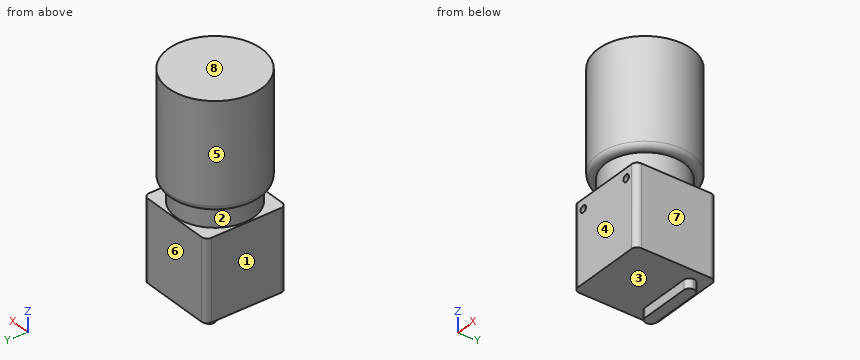
```python
from build123d import *

# Parameters (mm, degrees)
SKETCH_1_W             = 29
SKETCH_1_H             = 29
EXTRUDE_1_DEPTH        = 29
SKETCH_2_R             = 14
EXTRUDE_2_DEPTH        = 7.2
HOLE_WIZARD_M3_1_D     = 2.5
HOLE_WIZARD_M3_1_DEPTH = 7.5
HOLE_WIZARD_M3_1_TIP   = 0.751075774
SKETCH_6_R             = 16.75
EXTRUDE_3_DEPTH        = 38
FILLET_1_R             = 2
SKETCH_7_W             = 22
SKETCH_7_H             = 4
EXTRUDE_4_DEPTH        = 3.5
FILLET_2_R             = 2


with BuildPart() as part:
    # 草图1 → 凸台-拉伸1 (new body)
    with BuildSketch(Plane.XY):
        Rectangle(SKETCH_1_W, SKETCH_1_H)
    extrude(amount=EXTRUDE_1_DEPTH)

    # 草图2 → 凸台-拉伸2 (add)
    with BuildSketch(Plane.XY.offset(29)):
        Circle(SKETCH_2_R)
    extrude(amount=EXTRUDE_2_DEPTH)

    # M3 螺纹孔1
    with Locations(Plane(origin=(0, -14.5, 0), x_dir=(-1, 0, 0), z_dir=(0, -1, 0))):
        with Locations((10, -25.5), (-10, -25.5)):
            Hole(HOLE_WIZARD_M3_1_D / 2, depth=HOLE_WIZARD_M3_1_DEPTH)
            with Locations((0, 0, -(HOLE_WIZARD_M3_1_DEPTH + HOLE_WIZARD_M3_1_TIP / 2))):  # 118° drill point
                Cone(0, HOLE_WIZARD_M3_1_D / 2, HOLE_WIZARD_M3_1_TIP, mode=Mode.SUBTRACT)

    # 草图6 → 凸台-拉伸3 (add)
    with BuildSketch(Plane.XY.offset(36.2)):
        Circle(SKETCH_6_R)
    extrude(amount=EXTRUDE_3_DEPTH)

    # 圆角1
    fillet_1_edges = [part.edges().sort_by_distance(p)[0] for p in [
        (-16.75, 0, 36.2),
        (-14.5, 14.5, 14.5),
        (14.5, 14.5, 14.5),
        (14.5, -14.5, 14.5),
        (-14.5, -14.5, 14.5),
    ]]
    fillet(fillet_1_edges, radius=FILLET_1_R)

    # 草图7 → 凸台-拉伸4 (add)
    with BuildSketch(Plane(origin=(0, 0, 0), x_dir=(-1, 0, 0), z_dir=(0, 0, -1))):
        with Locations((0, 9)):
            Rectangle(SKETCH_7_W, SKETCH_7_H)
    extrude(amount=EXTRUDE_4_DEPTH)

    # 圆角2
    fillet_2_edges = [part.edges().sort_by_distance(p)[0] for p in [
        (-11, 7, -1.75),
        (-11, 11, -1.75),
        (11, 7, -1.75),
        (11, 11, -1.75),
    ]]
    fillet(fillet_2_edges, radius=FILLET_2_R - 0.0001)  # a hair under: the kernel refuses the full size


solid = part.part
```
The model under review builds one solid part; all positions refer to its coordinate system, in mm. Face numbers are marked on the shaded views. A direction names the side the tool comes from. Give positions to 0.01 mm unless a question says otherwise; leave off trailing zeros. Write each loop counter-clockwise with the first axis right and the second up, starting at its lowest first coordinate (ties: lowest second). Pieces come first, ordered by that corner, then holes. Notation, with made-up numbers: M 9,41 L 56,41 A18 cw 56,63 Z; hole C 77.25,-13 d5. An arc over 180 degrees is marked long. Write item = value, one per line. Start each with the question number.
Q1. We need section B-B (z = 23.5). State the section outline as (x, y) points, plus the area to 3 significant figures.
Q2. We need section A-A (y = 0). State the section outline as (x, z) points.
Q3. Mouldability with a two-part tool opening along Z and no side actions: class the marked faces 1, 2 and 3 as released by +Z, released by -Z, zero draft, split by the parting line, or undercut.
Q4. We need section C-C (x = 0). State the section outline as (y, z) points, plus the area to 3 significant figures.
Q5. Clearance check with flat-ended pins moving along their axes: pin 1 (3 mm diameter, centred on y = -12.5, z = 50.5, fed in from -X); pin 2 (6 mm diameter, centred on x = -12.5, z = 38.5, fed in from -Y); pin 3 (12.5 mm diameter, centred on x = 3, z = 11.5, fed in from +Y). State where each tip first meets the part, or that it passes through.
Q6. For line 1 (X direction, y = -8.5, z = 25.5); line 2 (Z direction, x = -10, y = -10); line 3 (Z direction, x = -10, y = -9), list the stretches that pass through material, from the lowest coordinate up.
Q7. We need section D-D (y = -8). Give the number of separate pieces and of enclosed holes in the cut face, plus the area to 3 significant figures.
Q8. Machinability: for the marked faces 4, 5, 6, 7 and 8, which of the approach directions +Z, -Z, +X, -X, +Y, -Y give a long, thin tool a straight path to every point of the face, cutting with its end or side? Answer none if there is none.
Result set:
q1.outline = M -14.5,-12.5 A2 ccw -12.5,-14.5 L 12.5,-14.5 A2 ccw 14.5,-12.5 L 14.5,12.5 A2 ccw 12.5,14.5 L -12.5,14.5 A2 ccw -14.5,12.5 Z
q1.area = 838 mm2
q2.outline = M -16.75,38.2 A2 ccw -14.75,36.2 L -14,36.2 L -14,29 L -14.5,29 L -14.5,0 L 14.5,0 L 14.5,29 L 14,29 L 14,36.2 L 14.75,36.2 A2 ccw 16.75,38.2 L 16.75,74.2 L -16.75,74.2 Z
q3.face_1 = zero draft
q3.face_2 = undercut
q3.face_3 = released by -Z
q4.outline = M -16.75,38.2 A2 ccw -14.75,36.2 L -14,36.2 L -14,29 L -14.5,29 L -14.5,0 L 7,0 L 7,-3.5 L 11,-3.5 L 11,0 L 14.5,0 L 14.5,29 L 14,29 L 14,36.2 L 14.75,36.2 A2 ccw 16.75,38.2 L 16.75,74.2 L -16.75,74.2 Z
q4.area = 2,330 mm2
q5.pin_1 = -12.63
q5.pin_2 = -13.8
q5.pin_3 = 14.5
q6.line_1 = -14.5 to -11.25, -8.75 to 8.75, 11.25 to 14.5
q6.line_2 = 0 to 24.25, 26.75 to 29, 36.2 to 74.2
q6.line_3 = 0 to 24.25, 26.75 to 74.2
q7.separate_pieces = 1
q7.enclosed_holes = 2
q7.area = 2,110 mm2
q8.face_4 = -Z, +X, -X, -Y
q8.face_5 = +Z
q8.face_6 = -Z, +X, -X, +Y
q8.face_7 = -Z, +X, +Y, -Y
q8.face_8 = +Z, +X, -X, +Y, -Y
